Verification items for the finished model (mm, model axes). A direction names the side the tool comes from. Coordinates: 2 decimals unless noted, no trailing zeros. Order: outer loops, then holes, each group sorted by start corner. A loop starts at its lowest first (then second) coordinate and runs counter-clockwise, first axis right, second up. Notation, with made-up numbers: M 70,-32 L 86,-32 A12 cw 86,-22 Z; hole C 16,19 d4. An arc over 180 degrees is marked long. Use one line per item in the form item = value. Start each with the question number.
```python
from build123d import *

# Parameters (mm, degrees)
CROQUIS1_W              = 2.5
CROQUIS1_H              = 13.5
SALIENTE_EXTRUIR1_DEPTH = 3
CROQUIS2_W              = 3.5
CROQUIS2_H              = 2
SALIENTE_EXTRUIR2_DEPTH = 9
CROQUIS3_R              = 1.125
CORTAR_EXTRUIR1_DEPTH   = 13
CROQUIS5_W              = 2
CROQUIS5_H              = 4
SALIENTE_EXTRUIR3_DEPTH = 4
CROQUIS6_R              = 1.125
CORTAR_EXTRUIR3_DEPTH   = 23.299103121
REDONDEO2_R             = 1


with BuildPart() as part:
    # Croquis1 → Saliente-Extruir1 (new body)
    with BuildSketch(Plane(origin=(0, 0, 0), x_dir=(1, 0, 0), z_dir=(0, 1, 0))):
        with BuildLine():
            Line((-2, -10), (2, -10))
            ThreePointArc((2, -10), (4.121320344, -9.121320344), (5, -7))
            Line((5, -7), (5, 7))
            ThreePointArc((5, 7), (4.121320344, 9.121320344), (2, 10))
            Line((2, 10), (-2, 10))
            ThreePointArc((-2, 10), (-4.121320344, 9.121320344), (-5, 7))
            Line((-5, 7), (-5, -7))
            ThreePointArc((-5, -7), (-4.121320344, -9.121320344), (-2, -10))
        make_face()
        Rectangle(CROQUIS1_W, CROQUIS1_H, mode=Mode.SUBTRACT)
    extrude(amount=SALIENTE_EXTRUIR1_DEPTH)

    # Croquis2 → Saliente-Extruir2 (add)
    with BuildSketch(Plane(origin=(0, 3, 0), x_dir=(1, 0, 0), z_dir=(0, 1, 0))):
        with Locations((-3.25, 5.5)):
            Rectangle(CROQUIS2_W, CROQUIS2_H)
        with Locations((-3.25, -5.5)):
            Rectangle(CROQUIS2_W, CROQUIS2_H)
        with Locations((3.25, -5.5)):
            Rectangle(CROQUIS2_W, CROQUIS2_H)
    extrude(amount=SALIENTE_EXTRUIR2_DEPTH)

    # Croquis3 → Cortar-Extruir1 (cut)
    with BuildSketch(Plane.XY.offset(6.5)):
        with Locations((3.5, 10)):
            Circle(CROQUIS3_R)
    extrude(amount=-CORTAR_EXTRUIR1_DEPTH, mode=Mode.SUBTRACT)

    # Croquis5 → Saliente-Extruir3 (add)
    with BuildSketch(Plane.ZY.offset(5)):
        with Locations((5.5, 10)):
            Rectangle(CROQUIS5_W, CROQUIS5_H)
        with Locations((-5.5, 10)):
            Rectangle(CROQUIS5_W, CROQUIS5_H)
    extrude(amount=SALIENTE_EXTRUIR3_DEPTH)

    # Croquis6 → Cortar-Extruir3 (cut, through all)
    with BuildSketch(Plane.XY.offset(6.5)):
        with Locations((-7, 10)):
            Circle(CROQUIS6_R)
    extrude(amount=-CORTAR_EXTRUIR3_DEPTH, mode=Mode.SUBTRACT)

    # Redondeo2
    redondeo2_edges = [part.edges().sort_by_distance(p)[0] for p in [
        (-1.5, 12, -5.5),
        (-1.5, 12, 5.5),
        (1.5, 12, 5.5),
        (5, 12, 5.5),
        (-9, 8, 5.5),
        (-9, 12, 5.5),
        (-9, 12, -5.5),
        (-9, 8, -5.5),
    ]]
    fillet(redondeo2_edges, radius=REDONDEO2_R)


solid = part.part
```
1. Cross-section at C-C on y = 1.5. Enter the section's corners in (x, z), and give its area (3 significant figures).
2. Cross-section at D-D on y = 10. Enter the section's corners in (x, z) (3 decimals).
3. Cross-section at A-A on z = 4.25. Enter the section's corners in (x, y), and give its area (3 significant figures).
4. Cross-section at B-B on x = -7. Enter the section's corners in (y, z) (3 decimals), and give its area (3 significant figures).
5. Depth check by flat-ended pin: P1, Ø4, axis at y = 6.5, z = -3, coming from the +X side; P2, Ø1, axis at x = 2.5, y = 7, coming from the +Z side; P3, Ø1, axis at y = 6, z = 6, coming from the -X side; P4, Ø1, axis at y = 4, z = 3, coming from the +X side. Enter the tip coordinate at first touch or a pass-through.
6. Material ranges on line 1 along Y through (x, z) = (3.5, 5.3) (3 decimals); line 2 along Y through (x, z) = (-7, 5.7) (3 decimals); line 3 along X through (y, z) = (5.5, 5.25), recorded low to high.
7. Release check for a two-part mould opening along Y. For faces 1 (the cylindrical face through (-1.785, 11.699, -5.514)), 2 (the flat face through (-6, 8, 5)), 3 (the flat face through (0, 1, -10)), 4 (the cylindrical face through (-6.481, 9.002, 5.514)) record: pulls with the +Y half, pulls with the -Y half, needs draft (parallel to the pull), parting line crosses it, or undercut.
8. Tool access check on faces 5 (the flat face through (-4, 8, 4.5)), 6 (the flat face through (0, 1, -6.75)), 7 (the cylindrical face through (4.1, 1.48, 9.14)), 8 (the flat face through (-6, 8, -6)), 9 (the flat face through (-4, 8, 6.5)). Record the directions out of +Z, -Z, +X, -X, +Y, -Y that give a thin tool (end or side, any length) a straight path to the whole face; none if there is none.
Final values:
q1.outline = M -5,-7 A3 ccw -2,-10 L 2,-10 A3 ccw 5,-7 L 5,7 A3 ccw 2,10 L -2,10 A3 ccw -5,7 Z; hole M -1.25,-6.75 L 1.25,-6.75 L 1.25,6.75 L -1.25,6.75 Z
q1.area = 159 mm2
q2.outline = M -9,-6.5 L -8.125,-6.5 L -8.125,-4.5 L -9,-4.5 Z; M -9,4.5 L -8.125,4.5 L -8.125,6.5 L -9,6.5 Z; M -5.875,-6.5 L -1.5,-6.5 L -1.5,-4.5 L -5.875,-4.5 Z; M -5.875,4.5 L -1.5,4.5 L -1.5,6.5 L -5.875,6.5 Z; M 1.5,4.5 L 2.375,4.5 L 2.375,6.5 L 1.5,6.5 Z; M 4.625,4.5 L 5,4.5 L 5,6.5 L 4.625,6.5 Z
q3.outline = M -5,0 L -1.25,0 L -1.25,3 L -5,3 Z; M 1.25,0 L 5,0 L 5,3 L 1.25,3 Z
q3.area = 22.5 mm2
q4.outline = M 8,-6.5 L 8.875,-6.5 L 8.875,-4.5 L 8,-4.5 Z; M 8,4.5 L 8.875,4.5 L 8.875,6.5 L 8,6.5 Z; M 11.125,-6.5 L 12,-6.5 L 12,-4.5 L 11.125,-4.5 Z; M 11.125,4.5 L 12,4.5 L 12,6.5 L 11.125,6.5 Z
q4.area = 7.00 mm2
q5.P1 = -1.5
q5.P2 = 6.5
q5.P3 = -5
q5.P4 = through
q6.line_1 = 0 to 8.875, 11.125 to 12
q6.line_2 = 8 to 8.875, 11.125 to 12
q6.line_3 = -5 to -1.5, 1.5 to 5
q7.face_1 = pulls with the +Y half
q7.face_2 = pulls with the -Y half
q7.face_3 = needs draft
q7.face_4 = undercut
q8.face_5 = +X, -X, +Y
q8.face_6 = +Y, -Y
q8.face_7 = +Z, +X, +Y, -Y
q8.face_8 = +Z, -Z, -X, -Y
q8.face_9 = +Z, +X, -X, +Y
